Could you check a few things on this model? Use its own coordinates, in mm. A direction names the side the tool comes from. Round coordinates to 2 decimals unless told otherwise and drop trailing zeros. Loops run counter-clockwise (first coordinate to the right, second up) from the corner with the lowest first, then second, coordinate; pieces in that order, holes last. Notation, with made-up numbers: M 68.5,4.5 L 73.5,4.5 A15 ccw 73.5,16.5 Z; hole C 78,48 d2. An arc over 180 degrees is marked long. Answer in a Markdown table with one row per item.
```python
from build123d import *

# Parameters (mm, degrees)
SKETCH_1_W          = 103
SKETCH_1_H          = 90.5
EXTRUDE_1_DEPTH     = 35
CUT_EXTRUDE_1_DEPTH = 30
SKETCH_3_W          = 84.803967954
SKETCH_3_H          = 48.355269134
CUT_EXTRUDE_2_DEPTH = 30


with BuildPart() as part:
    # 草图1 → 凸台-拉伸1 (new body)
    with BuildSketch(Plane.XY):
        with Locations((51.5, 45.25)):
            Rectangle(SKETCH_1_W, SKETCH_1_H)
    extrude(amount=EXTRUDE_1_DEPTH)

    # 草图2 → 切除-拉伸1 (cut)
    with BuildSketch(Plane.XY.offset(35)):
        Polygon((0, 32.144730866), (0, 0), (3.691599488, 0), (3.691599488, 9.794798376), (9.000778853, 9.794798376), (9.000778853, 0), (14.053062443, 0), (14.053062443, 14.162026564), (33.5771414, 14.162026564), (33.5771414, 0), (38.80068884, 0), (38.80068884, 18.272358976), (51.988005329, 18.272358976), (51.988005329, 0), (56.869025068, 0), (56.869025068, 18.0154632), (69.028758454, 18.0154632), (69.028758454, 0), (73.652882417, 0), (73.652882417, 24.86601722), (90.351107841, 24.86601722), (90.351107841, 0), (92.491905972, 0), (92.491905972, 8.253423721), (99.085564217, 8.253423721), (99.085564217, 0), (103, 0), (103, 24.86601722), (94.803967954, 24.86601722), (94.803967954, 32.144730866), align=None)
    extrude(amount=-CUT_EXTRUDE_1_DEPTH, mode=Mode.SUBTRACT)

    # 草图3 → 切除-拉伸2 (cut)
    with BuildSketch(Plane.XY.offset(35)):
        Polygon((0, 90.5), (0, 32.144730866), (94.803967954, 32.144730866), (94.803967954, 80.939676354), (103, 80.939676354), (103, 90.5), align=None)
        with Locations((47.401983977, 61.322365433)):
            Rectangle(SKETCH_3_W, SKETCH_3_H, mode=Mode.SUBTRACT)
    extrude(amount=-CUT_EXTRUDE_2_DEPTH, mode=Mode.SUBTRACT)


solid = part.part
```
1) I want a section at A-A, the plane z = 18. State how many separate pieces and enclosed holes the cut face has, plus the area to 3 significant figures.
Computed:
| item | result |
|---|---|
| separate pieces | 8 |
| enclosed holes | 0 |
| area | 5,820 mm² |
2) I need wall thicknesses on line 1 (Y direction, x = 39.5, z = 10); line 2 (X direction, y = 80, z = 27); line 3 (Y direction, x = 29, z = 22). Which ranges of each line are inside material? Lowest first, please.
Computed:
| item | result |
|---|---|
| line 1 | y = 0 to 18.27, 37.14 to 85.5 |
| line 2 | x = 5 to 89.8, 94.8 to 103 |
| line 3 | y = 0 to 14.16, 37.14 to 85.5 |
3) If we mould it in two halves opening along X, with no side actions, what happens to faces 5 (the face through (45, 18.272, 20)), 6 (the face through (0, 45, 2)), 7 (the face through (56.869, 9, 20))? For each: released by +X, released by -X, zero draft, split by the parting line, or undercut.
Computed:
| item | result |
|---|---|
| face 5 | zero draft |
| face 6 | released by -X |
| face 7 | undercut |
4) Which directions (+Z, -Z, +X, -X, +Y, -Y) give clear straight access to the entire face, cutting with the end or side of a thin tool? Please do faces 1 (the face through (6, 9.795, 20)), 2 (the face through (5, 61, 20)), 3 (the face through (89.804, 61, 20)), 4 (the face through (51.988, 9, 20)).
Computed:
| item | result |
|---|---|
| face 1 | +Z, -X |
| face 2 | +Z, -X, +Y |
| face 3 | +Z, +Y |
| face 4 | +Z, -Y |
5) Will these pins go through, and if not, where does the flat tip stop? P1, Ø13.5, axis at x = 82.5, z = 21.5, coming from the +Y side; P2, Ø10, axis at x = 81.5, y = 32, coming from the +Z side; P3, Ø5, axis at y = 10.5, z = 28.5, coming from the -X side.
Computed:
| item | result |
|---|---|
| P1 | stops at y = 85.5 |
| P2 | stops at z = 5 |
| P3 | stops at x = 3.69 |
6) I want a section at B-B, the plane y = 75. Please give me the cut outline in (x, z).
Computed:
| item | result |
|---|---|
| outline | M 0,0 L 103,0 L 103,35 L 94.8,35 L 94.8,5 L 89.8,5 L 89.8,35 L 5,35 L 5,5 L 0,5 Z |
7) I want a section at C-C, the plane x = 65.5. Please give me the cut outline in (y, z), plus the area to 3 significant figures.
Computed:
| item | result |
|---|---|
| outline | M 0,0 L 90.5,0 L 90.5,5 L 85.5,5 L 85.5,35 L 37.14,35 L 37.14,5 L 18.02,5 L 18.02,35 L 0,35 Z |
| area | 2,440 mm² |
